```python
from build123d import *

# Parameters (mm, degrees)
F1_DEPTH = 8
F2_W     = 350
F2_H     = 358
F3_DEPTH = 8


with BuildPart() as f1:
    # F0 (on Top) → F1 (new body)
    with BuildSketch(Plane.XY):
        with BuildLine():
            Line((350, 0), (0, 0))
            Line((0, 0), (0, -350))
            Line((0, -350), (350, -350))
            Line((350, -350), (350, -200))
            Line((350, -200), (300, -200))
            Line((300, -200), (286.824584, -200))
            ThreePointArc((286.824584, -200), (90, -175), (286.824584, -150))
            Line((286.824584, -150), (300, -150))
            Line((300, -150), (350, -150))
            Line((350, -150), (350, 0))
        make_face()
    extrude(amount=F1_DEPTH)

    # F2 (on Right) → F3 (join)
    with BuildSketch(Plane.YZ):
        with Locations((-175, 179)):
            Rectangle(F2_W, F2_H)
    extrude(amount=F3_DEPTH)


solid = f1.part
```
Build history of the part. All positions in model axes, mm. A direction names the side the tool comes from. Coordinates: 2 decimals unless noted, no trailing zeros. Order: outer loops, then holes, each group sorted by start corner. A loop starts at its lowest first (then second) coordinate and runs counter-clockwise, first axis right, second up.
Item 1: Mould opens along Y. For faces 1 (the flat face through (6, -350, 99)), 2 (the cylindrical face through (90.08, -179.04, 3.94)), 3 (the flat face through (8, -177, 185)) say: released by +Y, released by -Y, zero draft, split by the parting line, or undercut.
Filled in:
face 1: released by -Y
face 2: undercut
face 3: zero draft
Item 2: Drill centre lines: L1, parallel to Y at x = 190, z = 1.5; L2, parallel to Z at x = 242.5, y = -42; L3, parallel to X at y = -175, z = 2. Where is each one in solid material? Low to high.
Filled in:
L1: y = -350 to -275, -75 to 0
L2: z = 0 to 8
L3: x = 0 to 90
Item 3: Saw through at C-C on y = -175. List the corners of the cut face in (x, z).
Filled in:
outline: (0, 0) - (90, 0) - (90, 8) - (8, 8) - (8, 358) - (0, 358) - close
Item 4: Saw through at B-B on y = -214. List the corners of the cut face in (x, z).
Filled in:
outline: (0, 0) - (97.92, 0) - (97.92, 8) - (8, 8) - (8, 358) - (0, 358) - close; (282.08, 0) - (350, 0) - (350, 8) - (282.08, 8) - close
Item 5: Saw through at A-A on x = 190. List the corners of the cut face in (y, z), then the cut area to 3 significant figures.
Filled in:
outline: (-350, 0) - (-275, 0) - (-275, 8) - (-350, 8) - close; (-75, 0) - (0, 0) - (0, 8) - (-75, 8) - close
area: 1,200 mm2
Item 6: Drop a flat-ended pin along its axis: pin 1 Ø10 at (y, z) = (-159.5, 255.5) entering from +X. Give the stop position or say it passes through.
Filled in:
pin 1: stops at x = 8
Item 7: Saw through at D-D on x = 321. List the corners of the cut face in (y, z).
Filled in:
outline: (-350, 0) - (-200, 0) - (-200, 8) - (-350, 8) - close; (-150, 0) - (0, 0) - (0, 8) - (-150, 8) - close
Item 8: Tool access for faces 4 (the flat face through (0, -173, 176)), 5 (the flat face through (101, -95, 8)): list every direction of +Z, -Z, +X, -X, +Y, -Y with a clear straight run to the whole face (end or side of a thin tool).
Filled in:
face 4: +Z, -Z, -X, +Y, -Y
face 5: +Z, +X, +Y, -Y
